```python
from build123d import *

# Parameters (mm, degrees)
F0_W     = 95.25
F0_H     = 63.5
F1_DEPTH = 25.4
F3_DEPTH = 25.401
F5_DEPTH = 63.501
F6_R     = 6.35
F7_DEPTH = 25.401
F9_DEPTH = 31.75


with BuildPart() as f1:
    # F0 (on Front) → F1 (new body)
    with BuildSketch(Plane.XZ):
        with Locations((47.625, 31.75)):
            Rectangle(F0_W, F0_H)
    extrude(amount=F1_DEPTH)

    # F2 (on face) → F3 (cut, through all)
    with BuildSketch(Plane.XZ.offset(25.4)):
        Polygon((95.25, 63.5), (50.8, 63.5), (95.25, 19.05), align=None)
    extrude(amount=-F3_DEPTH, mode=Mode.SUBTRACT)

    # F4 (on face) → F5 (cut, through all)
    with BuildSketch(Plane(origin=(0, 0, 0), x_dir=(1, 0, 0), z_dir=(0, 0, -1))):
        Polygon((95.25, 0), (95.25, 15.875), (79.375, 0), align=None)
    extrude(amount=-F5_DEPTH, mode=Mode.SUBTRACT)

    # F6 (on face) → F7 (cut, through all)
    with BuildSketch(Plane.XZ.offset(25.4)):
        with Locations((19.05, 50.8)):
            Circle(F6_R)
    extrude(amount=-F7_DEPTH, mode=Mode.SUBTRACT)

    # F8 (on face) → F9 (join)
    with BuildSketch(Plane.XZ.offset(25.4)):
        Polygon((0, 31.75), (0, 6.35), (6.35, 6.35), (6.35, 0), (44.45, 0), (44.45, 12.7), (57.15, 12.7), (57.15, 19.05), (44.45, 19.05), (44.45, 31.75), align=None)
    extrude(amount=F9_DEPTH)


solid = f1.part
```
For this review, take the finished solid that the model builds, in its own axes (mm). A direction names the side the tool comes from. Coordinates: 2 decimals unless noted, no trailing zeros. Loops run counter-clockwise (first coordinate to the right, second up) from the corner with the lowest first, then second, coordinate; pieces in that order, holes last.
1. Add section D-D, the plane z = 15.5. Give the boundary of the cut face in (x, y) (3 decimals), then the cut area to 3 significant figures.
2. Mouldability with a two-part tool opening along X and no side actions: class faces 1 (the flat face through (36, -22, 0)), 2 (the cylindrical face through (22.464, -12.878, 56.154)), 3 (the flat face through (57.15, -41, 16)) as +X half, -X half, draft (parallel to the pull), parting line (faces both ways), or undercut.
3. For line 1 (Z direction, x = 19.05, y = -14.75); line 2 (Y direction, x = 57, z = 32.5); line 3 (Z direction, x = 52, y = -42), list the stretches that pass through material, from the lowest coordinate up.
4. Insertion check: P1, Ø8, axis at y = -36, z = 38.5, coming from the +X side; P2, Ø12, axis at x = 74, z = 24, coming from the -Y side; P3, Ø1.9, axis at y = -40, z = 4, coming from the -X side; P4, Ø6.5, axis at x = 48, y = -41, coming from the +Z side. Each pin has a flat end and moves straight along its axis. Give the tip position at first contact, or say it passes through.
5. Add section A-A, the plane x = 19.05. Give the boundary of the cut face in (y, z), then the cut area to 3 significant figures.
6. Add section B-B, the plane z = 50.8. Give the boundary of the cut face in (x, y), then the cut area to 3 significant figures.
7. For faces 4 (the flat face through (23, -41, 31.75)), 5 (the flat face through (6.35, -41, 3)), 6 (the flat face through (44.45, -41, 25)), list the 3-axis set-ups (+Z, -Z, +X, -X, +Y, -Y) from which the entire face can be reached by the end or side of a thin tool; tool diameter is ignored.
8. Add section C-C, the plane y = -17.5. Give the boundary of the cut face in (x, z).
Result:
1. outline: (0, -57.15) - (57.15, -57.15) - (57.15, -25.4) - (95.25, -25.4) - (95.25, -15.875) - (79.375, 0) - (0, 0) - close
1. area: 4,110 mm2
2. face 1: draft
2. face 2: undercut
2. face 3: +X half
3. line 1: z = 0 to 44.45, 57.15 to 63.5
3. line 2: y = -25.4 to 0
3. line 3: z = 12.7 to 19.05
4. P1: passes through
4. P2: stops at y = -25.4
4. P3: stops at x = 6.35
4. P4: stops at z = 19.05
5. outline: (-57.15, 0) - (0, 0) - (0, 44.45) - (-25.4, 44.45) - (-25.4, 31.75) - (-57.15, 31.75) - close; (-25.4, 57.15) - (0, 57.15) - (0, 63.5) - (-25.4, 63.5) - close
5. area: 2,300 mm2
6. outline: (0, -25.4) - (12.7, -25.4) - (12.7, 0) - (0, 0) - close; (25.4, -25.4) - (63.5, -25.4) - (63.5, 0) - (25.4, 0) - close
6. area: 1,290 mm2
7. face 4: +Z, +X, -X, -Y
7. face 5: -Z, -X, -Y
7. face 6: +Z, +X, -Y
8. outline: (0, 0) - (95.25, 0) - (95.25, 19.05) - (50.8, 63.5) - (0, 63.5) - close; hole circle Ø12.7 at (19.05, 50.8)
